from build123d import *

# Parameters (mm, degrees)
SKETCH1_R               = 12
SKETCH1_R_2             = 6
BOSS_EXTRUDE1_DEPTH     = 10
SKETCH2_R               = 6
SKETCH2_R_2             = 12
BOSS_EXTRUDE3_DEPTH     = 10
BOSS_EXTRUDE4_DEPTH     = 26
CUT_EXTRUDE3_START      = -41
CUT_EXTRUDE3_DEPTH      = 41
CUT_EXTRUDE4_REACH      = 168.878
SKETCH7_R               = 6
SKETCH8_R               = 22
CUT_EXTRUDE5_DEPTH      = 26
BOSS_EXTRUDE5_DEPTH     = 3
CHAMFER1_SIZE           = 3
CUT_EXTRUDE7_DEPTH      = 172.13826848
CUT_EXTRUDE7_DEPTH_BACK = 172.13826848
SKETCH12_W              = 45
SKETCH12_H              = 36


with BuildPart() as part:
    # Sketch1 → Boss-Extrude1 (new body)
    with BuildSketch(Plane(origin=(0, 0, 0), x_dir=(1, 0, 0), z_dir=(0, 1, 0))):
        with Locations(Location((0, 0, 0), (0, 0, 270))):
            Circle(SKETCH1_R)
        with Locations(Location((0, 0, 0), (0, 0, 270))):
            Circle(SKETCH1_R_2, mode=Mode.SUBTRACT)
    extrude(amount=-BOSS_EXTRUDE1_DEPTH)

    # Sketch2 → Boss-Extrude3 (add)
    with BuildSketch(Plane(origin=(0, 0, 0), x_dir=(1, 0, 0), z_dir=(0, 1, 0))):
        with BuildLine():
            Line((-1.328372743, 18.953506954), (-200, 12))
            ThreePointArc((-200, 12), (-212, 0), (-200, -12))
            Line((-200, -12), (-1.328372743, -18.953506954))
            Line((-1.328372743, -18.953506954), (0, -19))
            ThreePointArc((0, -19), (19, 0), (0, 19))
            Line((0, 19), (-1.328372743, 18.953506954))
        make_face()
        with Locations(Location((-200, 0, 0), (0, 0, 270))):
            Circle(SKETCH2_R, mode=Mode.SUBTRACT)
        Circle(SKETCH2_R_2, mode=Mode.SUBTRACT)
    extrude(amount=-BOSS_EXTRUDE3_DEPTH)

    # Sketch3 → Boss-Extrude4 (add)
    with BuildSketch(Plane.XZ.offset(10)):
        with BuildLine():
            Line((-191.415216863, -12.30046741), (-11.76781879, -18.588126342))
            ThreePointArc((-11.76781879, -18.588126342), (-14.841660941, -16.239615159), (-17.45663787, -13.389017675))
            Line((-17.45663787, -13.389017675), (-186.984061419, -7.45555785))
            ThreePointArc((-186.984061419, -7.45555785), (-188.93130171, -10.123434109), (-191.415216863, -12.30046741))
        make_face()
        with BuildLine():
            Line((-186.984061419, 7.45555785), (-17.45663787, 13.389017675))
            ThreePointArc((-17.45663787, 13.389017675), (-14.841660941, 16.239615159), (-11.76781879, 18.588126342))
            Line((-11.76781879, 18.588126342), (-191.415216863, 12.30046741))
            ThreePointArc((-191.415216863, 12.30046741), (-188.93130171, 10.123434109), (-186.984061419, 7.45555785))
        make_face()
    extrude(amount=BOSS_EXTRUDE4_DEPTH)

    # Sketch6 → Cut-Extrude3 (cut)
    with BuildSketch(Plane.XZ.offset(36).offset(CUT_EXTRUDE3_START)):
        with BuildLine():
            Line((-200, 12), (-191.415216863, 12.30046741))
            Line((-191.415216863, 12.30046741), (-150.48066119, 13.733176858))
            ThreePointArc((-150.48066119, 13.733176858), (-163.741585855, 0), (-150.48066119, -13.733176858))
            Line((-150.48066119, -13.733176858), (-191.415216863, -12.30046741))
            Line((-191.415216863, -12.30046741), (-200, -12))
            ThreePointArc((-200, -12), (-212, 0), (-200, 12))
        make_face()
    extrude(amount=CUT_EXTRUDE3_DEPTH, mode=Mode.SUBTRACT)

    # Sketch7 → Cut-Extrude4 (cut, up to next)
    with BuildSketch(Plane.XZ.offset(10), mode=Mode.PRIVATE) as cut_extrude4_sk1:
        with Locations(Location((-150, 0, 0), (0, 0, 270))):
            Circle(SKETCH7_R)
    cut_extrude4_tool1 = extrude(cut_extrude4_sk1.sketch, amount=-CUT_EXTRUDE4_REACH, mode=Mode.PRIVATE) & part.part
    add(cut_extrude4_tool1.solids().sort_by_distance((-150, -10, 0))[0], mode=Mode.SUBTRACT)

    # Sketch8 → Cut-Extrude5 (cut)
    with BuildSketch(Plane(origin=(0, -36, 0), x_dir=(-1, 0, 0), z_dir=(0, -1, 0))):
        with Locations((150, 0)):
            Circle(SKETCH8_R)
    extrude(amount=-CUT_EXTRUDE5_DEPTH, mode=Mode.SUBTRACT)

    # Sketch10 → Boss-Extrude5 (add)
    with BuildSketch(Plane(origin=(-0.489400484, 0, -13.982870983), x_dir=(0.999388062160532, 0, -0.03497858217562234), z_dir=(0.03497858217562234, 0, 0.9993880621605321))):
        Polygon((-128.434604534, -26), (-16.977626637, -26), (-16.977626637, -36), (-16.977626637, -46), (-128.434604534, -46), align=None)
    extrude(amount=BOSS_EXTRUDE5_DEPTH)

    # Chamfer1
    chamfer1_edges = [part.edges().sort_by_distance(p)[0] for p in [
        (-17.351702123, -36, -10.390853488),
        (-73.0460887, -46, -8.441549958),
        (-128.740475277, -36, -6.492246428),
    ]]
    chamfer(chamfer1_edges, length=CHAMFER1_SIZE - 0.0001)  # a hair under: the kernel refuses the full size

    # Sketch12 → Cut-Extrude7 (cut, two sides: drawn at the far end of the back side and taken through both)
    with BuildSketch(Plane.XY.offset(-CUT_EXTRUDE7_DEPTH_BACK)):
        with Locations((-110.810696752, -28)):
            Rectangle(SKETCH12_W, SKETCH12_H)
    extrude(amount=CUT_EXTRUDE7_DEPTH + CUT_EXTRUDE7_DEPTH_BACK, mode=Mode.SUBTRACT)


solid = part.part
Verification items for the finished model (mm, model axes). A direction names the side the tool comes from. Coordinates: 2 decimals unless noted, no trailing zeros. Order: outer loops, then holes, each group sorted by start corner. A loop starts at its lowest first (then second) coordinate and runs counter-clockwise, first axis right, second up. Notation, with made-up numbers: M -37.5,37.5 L -19.5,37.5 A20 cw -19.5,61.5 Z; hole C 12,53.25 d8. An arc over 180 degrees is marked long. One line per item, written item: value. Start each with the question number.
Item 1: Access from +Z, -Z, +X, -X, +Y, -Y to the whole of each face (thin tool, end or side, straight path). Record for faces 1 (the cylindrical face through (-14.882, -22.818, 16.203)), 2 (the flat face through (-51, -36, 15)), 3 (the flat face through (-88.311, -23, 13)).
Item 2: Gauge pin test, flat ends, axial feed: pin 1 (5 mm diameter, centred on x = -119.5, z = -7.5, fed in from -Y); pin 2 (10 mm diameter, centred on y = -22, z = 8.5, fed in from -X); pin 3 (2.5 mm diameter, centred on x = -48.5, z = -11.5, fed in from +Y); pin 4 (6 mm diameter, centred on x = -133, y = -8, fed in from -Z). Record the tip position at first contact, or that the pin passes through.
Item 3: Sectioned sample at D-D (y = -17). Enter the section's corners in (x, z).
Item 4: Sectioned sample at C-C (y = -4). Enter the section's corners in (x, z), then the cut area to 3 significant figures.
Item 5: Sectioned sample at B-B (z = 0). Enter the section's corners in (x, y), then the cut area to 3 significant figures.
Item 6: Mould release check, pull along Y, two halves, no side actions. Record for faces 4 (the flat face through (-53, -26, -11)), 5 (the flat face through (-51, -36, -15)), 6 (the cylindrical face through (19, -5, 0)): released by +Y, released by -Y, zero draft, split by the parting line, or undercut.
Item 7: Scan lines: probe 1 along X at (y, z) = (-6, 0); probe 2 along Y at (x, z) = (-96.5, 9); probe 3 along Y at (x, z) = (-45, -9.5). Record each from-to range of solid material in increasing order.
Conclusion:
1. face 1: +X, -Y
1. face 2: +Z, +X, -X, -Y
1. face 3: +Z, -Z, -X, -Y
2. pin 1: stops at y = -10
2. pin 2: stops at x = -88.31
2. pin 3: stops at y = 0
2. pin 4: stops at z = -14.45
3. outline: M -88.31,-15.91 L -11.77,-18.59 A22 cw -17.46,-13.39 L -88.31,-10.91 Z; M -88.31,10.91 L -17.46,13.39 A22 cw -11.77,18.59 L -88.31,15.91 Z
4. outline: M -150.48,-13.73 L 0,-19 A19 ccw 0,19 L -150.48,13.73 A13.74 ccw Z; hole C -150,0 d12; hole C 0,0 d12
4. area: 5,550 mm^2
5. outline: M -163.74,-10 L -156,-10 L -156,0 L -163.74,0 Z; M -144,-10 L -6,-10 L -6,0 L -144,0 Z; M 6,-10 L 19,-10 L 19,0 L 6,0 Z
5. area: 1,590 mm^2
6. face 4: undercut
6. face 5: released by -Y
6. face 6: zero draft
7. probe 1: x = -163.74 to -156, -144 to -6, 6 to 19
7. probe 2: y = -10 to 0
7. probe 3: y = -43.08 to -26, -10 to 0
